from build123d import *

# Parameters (mm, degrees)
EXTRUDE1_DEPTH     = 292.1
F_7060_LEFT_D      = 6.6548
F_7060_LEFT_DEPTH  = 20.1168
F_7060_LEFT_TIP    = 1.999303624
F_7060_RIGHT_D     = 6.6548
F_7060_RIGHT_DEPTH = 20.1168
F_7060_RIGHT_TIP   = 1.999303624


with BuildPart() as part:
    # Sketch1 → Extrude1 (new, symmetric)
    with BuildSketch(Plane.XY):
        with BuildLine():
            Line((-15.8242, 7.239), (-15.8242, 9.017))
            ThreePointArc((-15.8242, 9.017), (-15.452225612, 9.915025612), (-14.5542, 10.287))
            Line((-14.5542, 10.287), (-12.810497326, 10.287))
            ThreePointArc((-12.810497326, 10.287), (-12.470291755, 10.219328904), (-12.181879398, 10.026617928))
            Line((-12.181879398, 10.026617928), (-8.129198975, 5.973937506))
            ThreePointArc((-8.129198975, 5.973937506), (-7.09957176, 4.432991483), (-6.738014764, 2.615321716))
            Line((-6.738014764, 2.615321716), (-6.738014764, -2.615321716))
            ThreePointArc((-6.738014764, -2.615321716), (-7.09957176, -4.432991483), (-8.129198975, -5.973937506))
            Line((-8.129198975, -5.973937506), (-12.181879398, -10.026617928))
            ThreePointArc((-12.181879398, -10.026617928), (-12.470291755, -10.219328904), (-12.810497326, -10.287))
            Line((-12.810497326, -10.287), (-14.5542, -10.287))
            ThreePointArc((-14.5542, -10.287), (-15.452225612, -9.915025612), (-15.8242, -9.017))
            Line((-15.8242, -9.017), (-15.8242, -7.239))
            ThreePointArc((-15.8242, -7.239), (-15.712607684, -6.969592316), (-15.4432, -6.858))
            Line((-15.4432, -6.858), (-14.986, -6.858))
            Line((-14.986, -6.858), (-14.986, -5.6388))
            ThreePointArc((-14.986, -5.6388), (-15.447248241, -4.525248241), (-16.5608, -4.064))
            Line((-16.5608, -4.064), (-17.4752, -4.064))
            ThreePointArc((-17.4752, -4.064), (-18.588751759, -4.525248241), (-19.05, -5.6388))
            Line((-19.05, -5.6388), (-19.05, -15.875))
            ThreePointArc((-19.05, -15.875), (-18.12006403, -18.12006403), (-15.875, -19.05))
            Line((-15.875, -19.05), (15.875, -19.05))
            ThreePointArc((15.875, -19.05), (18.12006403, -18.12006403), (19.05, -15.875))
            Line((19.05, -15.875), (19.05, -5.6388))
            ThreePointArc((19.05, -5.6388), (18.588751759, -4.525248241), (17.4752, -4.064))
            Line((17.4752, -4.064), (16.5608, -4.064))
            ThreePointArc((16.5608, -4.064), (15.447248241, -4.525248241), (14.986, -5.6388))
            Line((14.986, -5.6388), (14.986, -6.858))
            Line((14.986, -6.858), (15.4432, -6.858))
            ThreePointArc((15.4432, -6.858), (15.712607684, -6.969592316), (15.8242, -7.239))
            Line((15.8242, -7.239), (15.8242, -9.017))
            ThreePointArc((15.8242, -9.017), (15.452225612, -9.915025612), (14.5542, -10.287))
            Line((14.5542, -10.287), (12.810497326, -10.287))
            ThreePointArc((12.810497326, -10.287), (12.470291755, -10.219328904), (12.181879398, -10.026617928))
            Line((12.181879398, -10.026617928), (8.129198975, -5.973937506))
            ThreePointArc((8.129198975, -5.973937506), (7.09957176, -4.432991483), (6.738014764, -2.615321716))
            Line((6.738014764, -2.615321716), (6.738014764, 2.615321716))
            ThreePointArc((6.738014764, 2.615321716), (7.09957176, 4.432991483), (8.129198975, 5.973937506))
            Line((8.129198975, 5.973937506), (12.181879398, 10.026617928))
            ThreePointArc((12.181879398, 10.026617928), (12.470291755, 10.219328904), (12.810497326, 10.287))
            Line((12.810497326, 10.287), (14.5542, 10.287))
            ThreePointArc((14.5542, 10.287), (15.452225612, 9.915025612), (15.8242, 9.017))
            Line((15.8242, 9.017), (15.8242, 7.239))
            ThreePointArc((15.8242, 7.239), (15.712607684, 6.969592316), (15.4432, 6.858))
            Line((15.4432, 6.858), (14.986, 6.858))
            Line((14.986, 6.858), (14.986, 5.6388))
            ThreePointArc((14.986, 5.6388), (15.447248241, 4.525248241), (16.5608, 4.064))
            Line((16.5608, 4.064), (17.4752, 4.064))
            ThreePointArc((17.4752, 4.064), (18.588751759, 4.525248241), (19.05, 5.6388))
            Line((19.05, 5.6388), (19.05, 15.875))
            ThreePointArc((19.05, 15.875), (18.12006403, 18.12006403), (15.875, 19.05))
            Line((15.875, 19.05), (5.6388, 19.05))
            ThreePointArc((5.6388, 19.05), (4.525248241, 18.588751759), (4.064, 17.4752))
            Line((4.064, 17.4752), (4.064, 16.5608))
            ThreePointArc((4.064, 16.5608), (4.525248241, 15.447248241), (5.6388, 14.986))
            Line((5.6388, 14.986), (6.858, 14.986))
            Line((6.858, 14.986), (6.858, 15.4432))
            ThreePointArc((6.858, 15.4432), (6.969592316, 15.712607684), (7.239, 15.8242))
            Line((7.239, 15.8242), (9.017, 15.8242))
            ThreePointArc((9.017, 15.8242), (9.915025612, 15.452225612), (10.287, 14.5542))
            Line((10.287, 14.5542), (10.287, 12.810497326))
            ThreePointArc((10.287, 12.810497326), (10.219328904, 12.470291755), (10.026617928, 12.181879398))
            Line((10.026617928, 12.181879398), (5.973937506, 8.129198975))
            ThreePointArc((5.973937506, 8.129198975), (4.432991483, 7.09957176), (2.615321716, 6.738014764))
            Line((2.615321716, 6.738014764), (-2.615321716, 6.738014764))
            ThreePointArc((-2.615321716, 6.738014764), (-4.432991483, 7.09957176), (-5.973937506, 8.129198975))
            Line((-5.973937506, 8.129198975), (-10.026617928, 12.181879398))
            ThreePointArc((-10.026617928, 12.181879398), (-10.219328904, 12.470291755), (-10.287, 12.810497326))
            Line((-10.287, 12.810497326), (-10.287, 14.5542))
            ThreePointArc((-10.287, 14.5542), (-9.915025612, 15.452225612), (-9.017, 15.8242))
            Line((-9.017, 15.8242), (-7.239, 15.8242))
            ThreePointArc((-7.239, 15.8242), (-6.969592316, 15.712607684), (-6.858, 15.4432))
            Line((-6.858, 15.4432), (-6.858, 14.986))
            Line((-6.858, 14.986), (-5.6388, 14.986))
            ThreePointArc((-5.6388, 14.986), (-4.525248241, 15.447248241), (-4.064, 16.5608))
            Line((-4.064, 16.5608), (-4.064, 17.4752))
            ThreePointArc((-4.064, 17.4752), (-4.525248241, 18.588751759), (-5.6388, 19.05))
            Line((-5.6388, 19.05), (-15.875, 19.05))
            ThreePointArc((-15.875, 19.05), (-18.12006403, 18.12006403), (-19.05, 15.875))
            Line((-19.05, 15.875), (-19.05, 5.6388))
            ThreePointArc((-19.05, 5.6388), (-18.588751759, 4.525248241), (-17.4752, 4.064))
            Line((-17.4752, 4.064), (-16.5608, 4.064))
            ThreePointArc((-16.5608, 4.064), (-15.447248241, 4.525248241), (-14.986, 5.6388))
            Line((-14.986, 5.6388), (-14.986, 6.858))
            Line((-14.986, 6.858), (-15.4432, 6.858))
            ThreePointArc((-15.4432, 6.858), (-15.712607684, 6.969592316), (-15.8242, 7.239))
        make_face()
        with BuildLine():
            Line((-2.615321716, -6.738014764), (2.615321716, -6.738014764))
            ThreePointArc((2.615321716, -6.738014764), (4.432991483, -7.09957176), (5.973937506, -8.129198975))
            Line((5.973937506, -8.129198975), (9.686553898, -11.841815367))
            ThreePointArc((9.686553898, -11.841815367), (9.93376449, -12.006996204), (10.225369265, -12.065))
            Line((10.225369265, -12.065), (16.51, -12.065))
            ThreePointArc((16.51, -12.065), (17.048815367, -12.288184633), (17.272, -12.827))
            Line((17.272, -12.827), (17.272, -14.478))
            ThreePointArc((17.272, -14.478), (16.453656347, -16.453656347), (14.478, -17.272))
            Line((14.478, -17.272), (-14.478, -17.272))
            ThreePointArc((-14.478, -17.272), (-16.453656347, -16.453656347), (-17.272, -14.478))
            Line((-17.272, -14.478), (-17.272, -12.827))
            ThreePointArc((-17.272, -12.827), (-17.048815367, -12.288184633), (-16.51, -12.065))
            Line((-16.51, -12.065), (-10.225369265, -12.065))
            ThreePointArc((-10.225369265, -12.065), (-9.93376449, -12.006996204), (-9.686553898, -11.841815367))
            Line((-9.686553898, -11.841815367), (-5.973937506, -8.129198975))
            ThreePointArc((-5.973937506, -8.129198975), (-4.432991483, -7.09957176), (-2.615321716, -6.738014764))
        make_face(mode=Mode.SUBTRACT)
        with BuildLine():
            Line((16.8656, 11.8618), (12.2428, 11.8618))
            ThreePointArc((12.2428, 11.8618), (11.973392316, 11.973392316), (11.8618, 12.2428))
            Line((11.8618, 12.2428), (11.8618, 16.8656))
            ThreePointArc((11.8618, 16.8656), (11.973392316, 17.135007684), (12.2428, 17.2466))
            Line((12.2428, 17.2466), (14.4526, 17.2466))
            ThreePointArc((14.4526, 17.2466), (16.428256347, 16.428256347), (17.2466, 14.4526))
            Line((17.2466, 14.4526), (17.2466, 12.2428))
            ThreePointArc((17.2466, 12.2428), (17.135007684, 11.973392316), (16.8656, 11.8618))
        make_face(mode=Mode.SUBTRACT)
        with BuildLine():
            Line((-11.8618, 16.8656), (-11.8618, 12.2428))
            ThreePointArc((-11.8618, 12.2428), (-11.973392316, 11.973392316), (-12.2428, 11.8618))
            Line((-12.2428, 11.8618), (-16.8656, 11.8618))
            ThreePointArc((-16.8656, 11.8618), (-17.135007684, 11.973392316), (-17.2466, 12.2428))
            Line((-17.2466, 12.2428), (-17.2466, 14.4526))
            ThreePointArc((-17.2466, 14.4526), (-16.428256347, 16.428256347), (-14.4526, 17.2466))
            Line((-14.4526, 17.2466), (-12.2428, 17.2466))
            ThreePointArc((-12.2428, 17.2466), (-11.973392316, 17.135007684), (-11.8618, 16.8656))
        make_face(mode=Mode.SUBTRACT)
        with BuildLine():
            Line((1.401430967, 3.017877069), (2.722376949, 4.338823051))
            ThreePointArc((2.722376949, 4.338823051), (4.338823051, 4.338823051), (4.338823051, 2.722376949))
            Line((4.338823051, 2.722376949), (3.017877069, 1.401430967))
            ThreePointArc((3.017877069, 1.401430967), (3.3274, 0), (3.017877069, -1.401430967))
            Line((3.017877069, -1.401430967), (4.338823051, -2.722376949))
            ThreePointArc((4.338823051, -2.722376949), (4.338823051, -4.338823051), (2.722376949, -4.338823051))
            Line((2.722376949, -4.338823051), (1.401430967, -3.017877069))
            ThreePointArc((1.401430967, -3.017877069), (0, -3.3274), (-1.401430967, -3.017877069))
            Line((-1.401430967, -3.017877069), (-2.722376949, -4.338823051))
            ThreePointArc((-2.722376949, -4.338823051), (-4.338823051, -4.338823051), (-4.338823051, -2.722376949))
            Line((-4.338823051, -2.722376949), (-3.017877069, -1.401430967))
            ThreePointArc((-3.017877069, -1.401430967), (-3.3274, 0), (-3.017877069, 1.401430967))
            Line((-3.017877069, 1.401430967), (-4.338823051, 2.722376949))
            ThreePointArc((-4.338823051, 2.722376949), (-4.338823051, 4.338823051), (-2.722376949, 4.338823051))
            Line((-2.722376949, 4.338823051), (-1.401430967, 3.017877069))
            ThreePointArc((-1.401430967, 3.017877069), (0, 3.3274), (1.401430967, 3.017877069))
        make_face(mode=Mode.SUBTRACT)
    extrude(amount=EXTRUDE1_DEPTH, both=True)

    # 7060-LEFT
    with Locations(Plane.XY.offset(292.1)):
        with Locations((0, 0)):
            Hole(F_7060_LEFT_D / 2, depth=F_7060_LEFT_DEPTH)
            with Locations((0, 0, -(F_7060_LEFT_DEPTH + F_7060_LEFT_TIP / 2))):  # 118° drill point
                Cone(0, F_7060_LEFT_D / 2, F_7060_LEFT_TIP, mode=Mode.SUBTRACT)

    # 7060-RIGHT
    with Locations(Plane(origin=(0, 0, -292.1), x_dir=(-1, 0, 0), z_dir=(0, 0, -1))):
        with Locations((0, 0)):
            Hole(F_7060_RIGHT_D / 2, depth=F_7060_RIGHT_DEPTH)
            with Locations((0, 0, -(F_7060_RIGHT_DEPTH + F_7060_RIGHT_TIP / 2))):  # 118° drill point
                Cone(0, F_7060_RIGHT_D / 2, F_7060_RIGHT_TIP, mode=Mode.SUBTRACT)


solid = part.part
Geometry check sheet. Reference: the model listing, model coordinates, mm. Round coordinates to 2 decimals unless told otherwise and drop trailing zeros.
Item 1: Mould release check, pull along Y, two halves, no side actions. Record for faces 1 (the flat face through (0, -19.05, 4)), 2 (the flat face through (-19.05, 11, 4)), 3 (the flat face through (0, -17.272, 4)): pulls with the +Y half, pulls with the -Y half, needs draft (parallel to the pull), parting line crosses it, or undercut.
Item 2: Cross-section at A-A on z = 75.5. Count the separate pieces of the cut face and the enclosed holes in it, then the cut area to 3 significant figures.
Item 3: Thickness scan on line 1 (Y direction, x = -6, z = 97); line 2 (X direction, y = 16, z = -194); line 3 (Y direction, x = -16, z = -227) (3 decimals). Record the ranges inside material, lowest first.
Item 4: Gauge pin test, flat ends, axial feed: pin 1 (2 mm diameter, centred on y = -2, z = 119, fed in from -X); pin 2 (1 mm diameter, centred on x = 17, z = -89, fed in from +Y); pin 3 (1 mm diameter, centred on y = 17, z = -123.5, fed in from -X). Record the tip position at first contact, or that the pin passes through.
Answer sheet:
1. face 1: pulls with the -Y half
1. face 2: needs draft
1. face 3: undercut
2. separate pieces: 1
2. enclosed holes: 4
2. area: 548 mm2
3. line 1: y = -19.05 to -17.27, -8.16 to 8.16, 14.99 to 19.05
3. line 2: x = -19.05 to -16.78, -11.86 to -4.17, 4.17 to 11.86, 16.78 to 19.05
3. line 3: y = -19.048 to -16.821, -12.065 to -4.167, 4.167 to 11.862, 16.779 to 19.048
4. pin 1: stops at x = -6.75
4. pin 2: stops at y = 18.99
4. pin 3: stops at x = -18.99
